Here's how the part is built. I have some questions about the finished solid (model axes, mm). Face numbers are marked on the shaded views. A direction names the side the tool comes from. Coordinates: 2 decimals unless noted, no trailing zeros. Write each loop counter-clockwise with the first axis right and the second up, starting at its lowest first coordinate (ties: lowest second). Pieces come first, ordered by that corner, then holes. Notation, with made-up numbers: (-23, 66) - (29, 66) arc R6 ccw to (29, 70) - close; hole circle Ø2 at (-20, 37). An arc over 180 degrees is marked (long way). Answer in a Markdown table with one row per item. Add a question column.
Item 1: Imagine slicing it at B-B (z = 41). Please give me the cut outline in (x, y).
Item 2: Imagine slicing it at C-C (z = 70.5). Please give me the cut outline in (x, y), plus the area to 3 significant figures.
Item 3: We'd pull the mould along X, two halves only. Please class the marked faces 4, 5, 6 and 7: +X half, -X half, draft (parallel to the pull), parting line (faces both ways), or undercut.
Item 4: Which directions (+Z, -Z, +X, -X, +Y, -Y) give clear straight access to the entire face, cutting with the end or side of a thin tool? Please do the marked faces 1, 2 and 3.
Item 5: I'm going to push flat-ended pins straight in: pin 1 (1.5 mm diameter, centred on x = -16.5, z = 57.5, fed in from +Y); pin 2 (21 mm diameter, centred on x = 21.5, y = -100, fed in from +Z); pin 3 (7.5 mm diameter, centred on x = 2, y = -25.5, fed in from -Z). Where does each tip first touch, or does it pass through?
Item 6: Imagine slicing it at A-A (y = -52.5). Please give me the cut outline in (x, z), plus the area to 3 significant figures.
Item 7: If I drill on probe 1 along Y at (x, z) = (33.5, 39); probe 2 along X at (y, z) = (-68, 31); probe 3 along Z at (x, y) = (27.5, -112), over which ranges is the centre line in solid material (lowest first)? Write a range as from..to.
from build123d import *

# Parameters (mm, degrees)
F1_DEPTH      = 38.1
F3_DEPTH      = 63.5
F3_DEPTH_BACK = 63.5
F5_DEPTH      = 273.05


with BuildPart() as f1:
    # F0 (on Front) → F1 (new body)
    with BuildSketch(Plane.XZ):
        with BuildLine():
            Line((-63.5, 50.8), (-63.5, 0))
            Line((-63.5, 0), (0, 0))
            Line((0, 0), (0, 63.5))
            ThreePointArc((0, 63.5), (-12.7, 76.2), (0, 88.9))
            Line((0, 88.9), (0, 101.6))
            ThreePointArc((0, 101.6), (-11.9529411765, 98.6117647059), (-21.0934256055, 90.3501730104))
            Line((-21.0934256055, 90.3501730104), (-47.625, 50.8))
            Line((-47.625, 50.8), (-63.5, 50.8))
        make_face()
        with BuildLine():
            Line((0, 63.5), (0, 0))
            Line((0, 0), (63.5, 0))
            Line((63.5, 0), (63.5, 50.8))
            Line((63.5, 50.8), (47.625, 50.8))
            Line((47.625, 50.8), (21.0934256055, 90.3501730104))
            ThreePointArc((21.0934256055, 90.3501730104), (11.9529411765, 98.6117647059), (0, 101.6))
            Line((0, 101.6), (0, 88.9))
            ThreePointArc((0, 88.9), (8.9802561211, 85.1802561211), (12.7, 76.2))
            ThreePointArc((12.7, 76.2), (8.9802561211, 67.2197438789), (0, 63.5))
        make_face()
    extrude(amount=F1_DEPTH)

    # F2 (on Right) → F3 (join, two sides)
    with BuildSketch(Plane.YZ) as f3_sk:
        Polygon((-304.8, 0), (0, 0), (0, 38.1), (-273.05, 38.1), (-273.05, 101.6), (-285.75, 101.6), (-304.8, 82.55), align=None)
    extrude(amount=-F3_DEPTH)
    extrude(f3_sk.sketch, amount=F3_DEPTH_BACK)

    # F4 (on Front) → F5 (cut)
    with BuildSketch(Plane.XZ):
        Polygon((-12.7, 16.51), (-12.7, 0), (12.7, 0), (12.7, 16.51), (31.75, 16.51), (31.75, 29.21), (12.7, 29.21), (12.7, 38.1), (-12.7, 38.1), (-12.7, 29.21), (-31.75, 29.21), (-31.75, 16.51), align=None)
    extrude(amount=F5_DEPTH, mode=Mode.SUBTRACT)


solid = f1.part
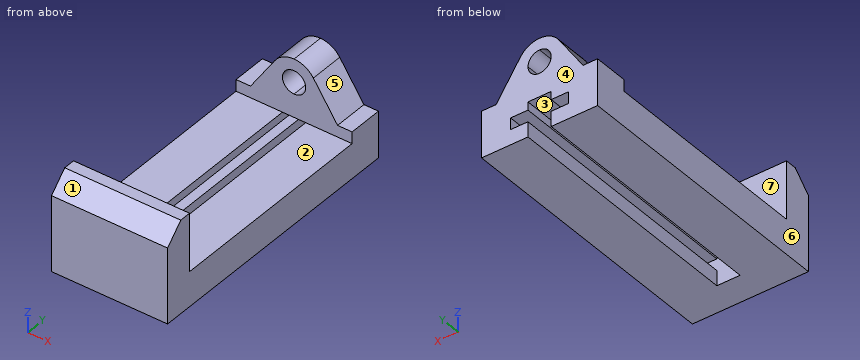
Here are the results:
| question | item | result |
|---|---|---|
| 1 | outline | (-63.5, -304.8) - (63.5, -304.8) - (63.5, -273.05) - (-63.5, -273.05) - close; (-63.5, -38.1) - (63.5, -38.1) - (63.5, 0) - (-63.5, 0) - close |
| 2 | outline | (-63.5, -304.8) - (63.5, -304.8) - (63.5, -273.05) - (-63.5, -273.05) - close; (-34.41, -38.1) - (-11.35, -38.1) - (-11.35, 0) - (-34.41, 0) - close; (11.35, -38.1) - (34.41, -38.1) - (34.41, 0) - (11.35, 0) - close |
| 2 | area | 5,790 mm2 |
| 3 | face 4 | draft |
| 3 | face 5 | +X half |
| 3 | face 6 | -X half |
| 3 | face 7 | undercut |
| 4 | face 1 | +Z, +X, -X, -Y |
| 4 | face 2 | +Z, +X, -X |
| 4 | face 3 | -Z, +Y |
| 5 | pin 1 | stops at y = 0 |
| 5 | pin 2 | stops at z = 38.1 |
| 5 | pin 3 | stops at z = 38.1 |
| 6 | outline | (-63.5, 0) - (-12.7, 0) - (-12.7, 16.51) - (-31.75, 16.51) - (-31.75, 29.21) - (-12.7, 29.21) - (-12.7, 38.1) - (-63.5, 38.1) - close; (12.7, 0) - (63.5, 0) - (63.5, 38.1) - (12.7, 38.1) - (12.7, 29.21) - (31.75, 29.21) - (31.75, 16.51) - (12.7, 16.51) - close |
| 6 | area | 3,390 mm2 |
| 7 | probe 1 | y = -304.8..-273.05, -38.1..0 |
| 7 | probe 2 | x = -63.5..-12.7, 12.7..63.5 |
| 7 | probe 3 | z = 0..16.51, 29.21..38.1 |
